The model under review builds one solid part; all positions refer to its coordinate system, in mm. Face numbers are marked on the shaded views. Round coordinates to 2 decimals unless told otherwise and drop trailing zeros. Order: outer loops, then holes, each group sorted by start corner. A loop starts at its lowest first (then second) coordinate and runs counter-clockwise, first axis right, second up. Notation, with made-up numbers: M 20.25,43.5 L 38.25,43.5 A32 cw 38.25,77.5 Z; hole C -13.75,-38.75 d10. An arc over 180 degrees is marked long. Use a Markdown table: item, result. Add a question column.
1. Consider section A-A on z = 6. Count the separate pieces of the cut face and the enclosed holes in it, then the cut area to 3 significant figures.
2. Consider section C-C on y = -40. State the section outline as (x, z) points, then the cut area to 3 significant figures.
3. Insertion check: P1, Ø2, axis at x = 3, y = -31, coming from the +Z side; P2, Ø3, axis at x = 34.5, y = 62, coming from the -Z side; P3, Ø1, axis at x = -36.5, z = 2, coming from the +Y side. Each pin has a flat end and moves straight along its axis. Give the tip position at first contact, or say it passes through.
4. To check wall thickness, follow probe 1 along Y at (x, z) = (34.5, 2); probe 2 along Y at (x, z) = (28, 3.25); probe 3 along X at (y, z) = (-15, 6.5). State the ranges of each line that lie inside material, in increasing order.
5. The part is to be moulded in two halves that separate along Y. For the marked faces 1, 2, 3 and 4, say which applies: +Y half, -Y half, draft (parallel to the pull), parting line (faces both ways), or undercut.
6. Consider section B-B on x = 28. State the section outline as (y, z) points.
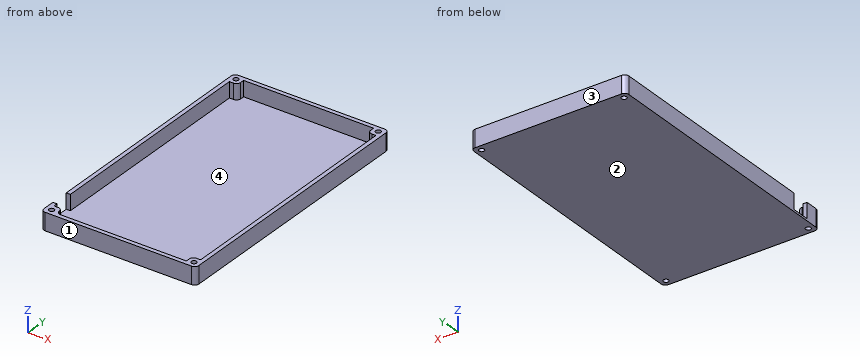
from build123d import *

# Parameters (mm, degrees)
F0_R     = 1.25
F0_W     = 2
F0_H     = 9
F1_DEPTH = 1
F2_DEPTH = 7.5
F3_R     = 1.99999


# Not quite as in the source:
# - a fillet or chamfer is up to 0.001 mm smaller than in the source, because OpenCascade refuses the exact size


with BuildPart() as f1:
    # F0 (on Top) → F1 (new body)
    with BuildSketch(Plane.XY):
        Polygon((-35.5, -48), (-35.5, 59), (-31.5, 59), (-31.5, 63), (31.5, 63), (31.5, 59), (35.5, 59), (35.5, -59), (31.5, -59), (31.5, -63), (-31.5, -63), (-31.5, -59), (-35.5, -59), (-35.5, -57), (-37.5, -57), (-37.5, -65), (37.5, -65), (37.5, 65), (-37.5, 65), (-37.5, -48), align=None)
        with Locations((-34.5, -62)):
            Circle(F0_R, mode=Mode.SUBTRACT)
        with Locations((34.5, -62)):
            Circle(F0_R, mode=Mode.SUBTRACT)
        with Locations((-34.5, 62)):
            Circle(F0_R, mode=Mode.SUBTRACT)
        with Locations((34.5, 62)):
            Circle(F0_R, mode=Mode.SUBTRACT)
        Polygon((-31.5, 59), (-35.5, 59), (-35.5, -48), (-35.5, -57), (-35.5, -59), (-31.5, -59), (-31.5, -63), (31.5, -63), (31.5, -59), (35.5, -59), (35.5, 59), (31.5, 59), (31.5, 63), (-31.5, 63), align=None)
        with Locations((-36.5, -52.5)):
            Rectangle(F0_W, F0_H)
    extrude(amount=-F1_DEPTH)

    # F0 (on Top) → F2 (join)
    with BuildSketch(Plane.XY):
        Polygon((-35.5, -48), (-35.5, 59), (-31.5, 59), (-31.5, 63), (31.5, 63), (31.5, 59), (35.5, 59), (35.5, -59), (31.5, -59), (31.5, -63), (-31.5, -63), (-31.5, -59), (-35.5, -59), (-35.5, -57), (-37.5, -57), (-37.5, -65), (37.5, -65), (37.5, 65), (-37.5, 65), (-37.5, -48), align=None)
        with Locations((-34.5, -62)):
            Circle(F0_R, mode=Mode.SUBTRACT)
        with Locations((34.5, -62)):
            Circle(F0_R, mode=Mode.SUBTRACT)
        with Locations((-34.5, 62)):
            Circle(F0_R, mode=Mode.SUBTRACT)
        with Locations((34.5, 62)):
            Circle(F0_R, mode=Mode.SUBTRACT)
    extrude(amount=F2_DEPTH)

    # F3 (radius 2 in the source; OpenCascade refuses exactly that, so slightly less here)
    f3_edges = [f1.edges().sort_by_distance(p)[0] for p in [
        (37.5, -65, 3.25),
        (37.5, 65, 3.25),
        (-37.5, 65, 3.25),
        (31.5, -59, 3.75),
        (-31.5, -63, 3.75),
        (-37.5, -65, 3.25),
        (-31.5, 59, 3.75),
        (31.5, 59, 3.75),
        (-31.5, -59, 3.75),
    ]]
    fillet(f3_edges, radius=F3_R)


solid = f1.part
Answer block:
| question | item | result |
|---|---|---|
| 1 | separate pieces | 1 |
| 1 | enclosed holes | 4 |
| 1 | area | 824 mm^2 |
| 2 | outline | M -37.5,-1 L 37.5,-1 L 37.5,7.5 L 35.5,7.5 L 35.5,0 L -35.5,0 L -35.5,7.5 L -37.5,7.5 Z |
| 2 | area | 105 mm^2 |
| 3 | P1 | z = 0 |
| 3 | P2 | z = -1 |
| 3 | P3 | y = 64.94 |
| 4 | probe 1 | -65 to -63.25, -60.75 to -59, 59 to 60.75, 63.25 to 65 |
| 4 | probe 2 | -65 to -63, 63 to 65 |
| 4 | probe 3 | -37.5 to -35.5, 35.5 to 37.5 |
| 5 | face 1 | -Y half |
| 5 | face 2 | draft |
| 5 | face 3 | +Y half |
| 5 | face 4 | undercut |
| 6 | outline | M -65,-1 L 65,-1 L 65,7.5 L 63,7.5 L 63,0 L -63,0 L -63,7.5 L -65,7.5 Z |
